Model file for the job. Use its own axes, mm. Give positions to 0.01 mm unless a question says otherwise; leave off trailing zeros. Order: outer loops, then holes, each group sorted by start corner. A loop starts at its lowest first (then second) coordinate and runs counter-clockwise, first axis right, second up. Notation, with made-up numbers: (-20.75, 55.5) -> (-16.75, 55.5) arc R27 cw to (-16.75, 90.5) -> close; hole circle Ø1 at (39, -17). An arc over 180 degrees is marked (long way). Use CSV: the item, a comma, the result in double quotes. Start each with the question number.
1. Cut at A-A on x = 0. List the corners of the cut face in (y, z), then the cut area to 3 significant figures.
2. Wall check: line 1 (Y direction, x = 0, z = 2.75); line 2 (Y direction, x = -4, z = 3.5); line 3 (Y direction, x = 8.25, z = 0.75). Give the ranges that are in metal, low to high. Write a range as from..to.
3. Cut at C-C on z = 4.25. List the corners of the cut face in (x, y).
4. Cut at D-D on x = 8. List the corners of the cut face in (y, z).
5. Pull direction X, two halves, no side cores. Call faces 1 (the cylindrical face through (-2.395, 19.875, 3.131)), 2 (the cylindrical face through (-13.97, 0.16, 3.13)), 3 (the flat face through (-9.4, -6.4, 6.35)): released by +X, released by -X, zero draft, split by the parting line, or undercut.
6. Drop flat-ended pins along their axis: pin 1 (1.5 mm diameter, centred on y = -28, z = 5.5, fed in from +X); pin 2 (2 mm diameter, centred on y = 7, z = 3.5, fed in from +X); pin 3 (4 mm diameter, centred on x = 10.5, y = -16.5, fed in from -Z). Give the stop position or say it passes through.
7. Cut at B-B on y = -35. List the corners of the cut face in (x, z), then the cut area to 3 significant figures.
```python
from build123d import *

# Parameters (mm, degrees)
F4_R     = 11.049
F5_DEPTH = 6.35


with BuildPart() as f5:
    # F4 (on Top) → F5 (new body)
    with BuildSketch(Plane.XY):
        with BuildLine():
            ThreePointArc((9.409508, 20.334971), (12.779118, 25.01674), (13.97, 30.660767))
            ThreePointArc((13.97, 30.660767), (-5.644027, 43.439885), (-9.409508, 20.334971))
            ThreePointArc((-9.409508, 20.334971), (0, 16.690767), (9.409508, 20.334971))
        make_face()
        with Locations((0, 30.660767)):
            Circle(F4_R, mode=Mode.SUBTRACT)
        with BuildLine():
            ThreePointArc((9.409508, 20.334971), (0, 16.690767), (-9.409508, 20.334971))
            ThreePointArc((-9.409508, 20.334971), (-7.199181, 15.330384), (-9.409508, 10.325796))
            ThreePointArc((-9.409508, 10.325796), (0, 13.97), (9.409508, 10.325796))
            ThreePointArc((9.409508, 10.325796), (7.199181, 15.330384), (9.409508, 20.334971))
        make_face()
        Circle(F4_R)
        with BuildLine():
            ThreePointArc((9.409508, 10.325796), (0, 13.97), (-9.409508, 10.325796))
            ThreePointArc((-9.409508, 10.325796), (-13.97, 0), (-9.409508, -10.325796))
            ThreePointArc((-9.409508, -10.325796), (0, -13.97), (9.409508, -10.325796))
            ThreePointArc((9.409508, -10.325796), (12.779118, -5.644027), (13.97, 0))
            ThreePointArc((13.97, 0), (12.779118, 5.644027), (9.409508, 10.325796))
        make_face()
        Circle(F4_R, mode=Mode.SUBTRACT)
        with BuildLine():
            ThreePointArc((9.409508, -10.325796), (0, -13.97), (-9.409508, -10.325796))
            ThreePointArc((-9.409508, -10.325796), (-7.199181, -15.330384), (-9.409508, -20.334971))
            ThreePointArc((-9.409508, -20.334971), (0, -16.690767), (9.409508, -20.334971))
            ThreePointArc((9.409508, -20.334971), (7.199181, -15.330384), (9.409508, -10.325796))
        make_face()
        with BuildLine():
            ThreePointArc((9.409508, -20.334971), (0, -16.690767), (-9.409508, -20.334971))
            ThreePointArc((-9.409508, -20.334971), (-5.644027, -43.439885), (13.97, -30.660767))
            ThreePointArc((13.97, -30.660767), (12.779118, -25.01674), (9.409508, -20.334971))
        make_face()
        with Locations((0, -30.271422)):
            Circle(F4_R, mode=Mode.SUBTRACT)
    extrude(amount=F5_DEPTH)


solid = f5.part
```
Verdict:
1,outline,"(-44.63, 0) -> (-41.32, 0) -> (-41.32, 6.35) -> (-44.63, 6.35) -> close; (-19.22, 0) -> (-11.05, 0) -> (-11.05, 6.35) -> (-19.22, 6.35) -> close; (11.05, 0) -> (19.61, 0) -> (19.61, 6.35) -> (11.05, 6.35) -> close; (41.71, 0) -> (44.63, 0) -> (44.63, 6.35) -> (41.71, 6.35) -> close"
1,area,"146 mm^2"
2,line 1,"-44.63..-41.32, -19.22..-11.05, 11.05..19.61, 41.71..44.63"
2,line 2,"-44.05..-40.57, -19.97..-10.3, 10.3..20.36, 40.96..44.05"
2,line 3,"-41.93..-37.62, -22.92..-18.95, -11.71..-7.35, 7.35..11.71, 18.95..23.31, 38.01..41.93"
3,outline,"(-9.41, -20.33) arc R13.97 ccw (long way) to (13.97, -30.66) arc R13.97 ccw to (9.41, -20.33) arc R6.77 cw to (9.41, -10.33) arc R13.97 ccw to (13.97, 0) arc R13.97 ccw to (9.41, 10.33) arc R6.77 cw to (9.41, 20.33) arc R13.97 ccw to (13.97, 30.66) arc R13.97 ccw (long way) to (-9.41, 20.33) arc R6.77 cw to (-9.41, 10.33) arc R13.97 ccw to (-9.41, -10.33) arc R6.77 cw to start; hole circle Ø22.1 at (0, -30.27); hole circle Ø22.1 at (0, 0); hole circle Ø22.1 at (0, 30.66)"
4,outline,"(-42.11, 0) -> (-37.89, 0) -> (-37.89, 6.35) -> (-42.11, 6.35) -> close; (-22.65, 0) -> (-18.52, 0) -> (-18.52, 6.35) -> (-22.65, 6.35) -> close; (-12.14, 0) -> (-7.62, 0) -> (-7.62, 6.35) -> (-12.14, 6.35) -> close; (7.62, 0) -> (12.14, 0) -> (12.14, 6.35) -> (7.62, 6.35) -> close; (18.52, 0) -> (23.04, 0) -> (23.04, 6.35) -> (18.52, 6.35) -> close; (38.28, 0) -> (42.11, 0) -> (42.11, 6.35) -> (38.28, 6.35) -> close"
5,face 1,"undercut"
5,face 2,"released by -X"
5,face 3,"zero draft"
6,pin 1,"x = 13.84"
6,pin 2,"x = 12.62"
6,pin 3,"through"
7,outline,"(-13.28, 0) -> (-9.99, 0) -> (-9.99, 6.35) -> (-13.28, 6.35) -> close; (9.99, 0) -> (13.28, 0) -> (13.28, 6.35) -> (9.99, 6.35) -> close"
7,area,"41.8 mm^2"
